Autodesk Inventor part; units mm, degrees
ref_plane "YZ Plane" through (0, 0, 0) normal (1, 0, 0) x (0, 1, 0)
ref_plane "XZ Plane" through (0, 0, 0) normal (0, 1, 0) x (-1, 0, 0)
ref_plane "XY Plane" through (0, 0, 0) normal (0, 0, 1) x (1, 0, 0)
sketch "Skizze1" plane through (0, 0, 0) normal (0, 0, 1) x (1, 0, 0)
  line L0 (-5.4, 0) -> (32.4, 0)
  line L1 (0, -3.95) -> (0, 23.7)
  line L2 (0, 0) -> (0, 19.75)
  line L3 (2, 19.75) -> (0, 19.75)
  arc A0 (2, 19.75) -> (22, 19.75) centre (12, 19.75) ccw
  line L4 (22, 19.75) -> (27, 19.75)
  line L5 (27, 19.75) -> (27, 17.5)
  line L6 (27, 17.5) -> (25, 17.5)
  line L7 (25, 17.5) -> (25, 0)
  line L8 (0, 0) -> (25, 0)
  dimension "d0" = 27
  dimension "d1" = 2
  dimension "d2" = 39.5
  dimension "d3" = 10
  dimension "d4" = 12
  dimension "d5" = 5
  dimension "d6" = 35
revolve "Umdrehung1" add sketch "Skizze1" angle 360 about axis through (-10, 0, 0) along (1, 0, 0)
sketch "Skizze2" plane through (0, 0, 0) normal (-1, 0, 0) x (0, 0, 1)
  point P0 (0, 0)
  point P1 (0, 0)
hole "Bohrung1" at (0, 0, 0) direction (1, 0, 0) diameter 3.242 depth 16 tip angle 118
properties part number "Brennersockel"
Here's how the part is built. I have some questions about the finished solid (model axes, mm). A direction names the side the tool comes from. Coordinates: 2 decimals unless noted, no trailing zeros. Order: outer loops, then holes, each group sorted by start corner. A loop starts at its lowest first (then second) coordinate and runs counter-clockwise, first axis right, second up. Notation, with made-up numbers: (9, 14.25) -> (34, 14.25) arc R15 cw to (34, 23.25) -> close; hole circle Ø8 at (6, -1). An arc over 180 degrees is marked (long way). Answer in a Markdown table with one row per item.
(1) On a 3-axis mill with a long thin cutter (end or side, diameter ignored), from which of +Z, -Z, +X, -X, +Y, -Y can I reach the whole of each face in a straight line? I mean faces 4 (the face through (8.112, 1.438, 0.748)), 5 (the face through (25, 0, 0)), 6 (the face through (0, 0, -4)). Say none if no direction works.
Answer key:
| item | result |
|---|---|
| face 4 | -X |
| face 5 | +X |
| face 6 | +Z, -Z, -X, +Y, -Y |
(2) Please list where these lines run through material, in increasing order: probe 1 along Z at (x, y) = (26.3, 0); probe 2 along Z at (x, y) = (8, 0); probe 3 along X at (y, z) = (2.5, -17).
Answer key:
| item | result |
|---|---|
| probe 1 | -19.75 to -17.5, 17.5 to 19.75 |
| probe 2 | -10.58 to -1.62, 1.62 to 10.58 |
| probe 3 | 0 to 2.34, 21.66 to 25 |
(3) I want a section at B-B on x = 8.5. List the corners of the cut face in (y, z) for me (1 decimal).
Answer key:
| item | result |
|---|---|
| outline | circle Ø20.8 at (0, 0); hole circle Ø3.2 at (0, 0) |
(4) I want a section at A-A on x = 3.75. List the corners of the cut face in (y, z) for me.
Answer key:
| item | result |
|---|---|
| outline | circle Ø28.2 at (0, 0); hole circle Ø3.24 at (0, 0) |
(5) I want a section at C-C on x = 19. List the corners of the cut face in (y, z) for me.
Answer key:
| item | result |
|---|---|
| outline | circle Ø25.22 at (0, 0) |
(6) Thinking about a two-plate mould opening in Z: for faces 1 (the face through (1, -14.6, -13.3)), 2 (the face through (27, -12, -13)), 3 (the face through (25.986, -13.887, 10.648)), which applies, +Z half, -Z half, draft (parallel to the pull), parting line (faces both ways), or undercut?
Answer key:
| item | result |
|---|---|
| face 1 | parting line |
| face 2 | draft |
| face 3 | undercut |
(7) Will these pins go through, and if not, where does the flat tip stop? pin 1 Ø3 at (y, z) = (-5.5, -13) entering from +X; pin 2 Ø10 at (x, y) = (19.5, 6.5) entering from -Z; pin 3 Ø12 at (x, y) = (14, -13) entering from -Z.
Answer key:
| item | result |
|---|---|
| pin 1 | x = 25 |
| pin 2 | z = -19.63 |
| pin 3 | z = -8.13 |
